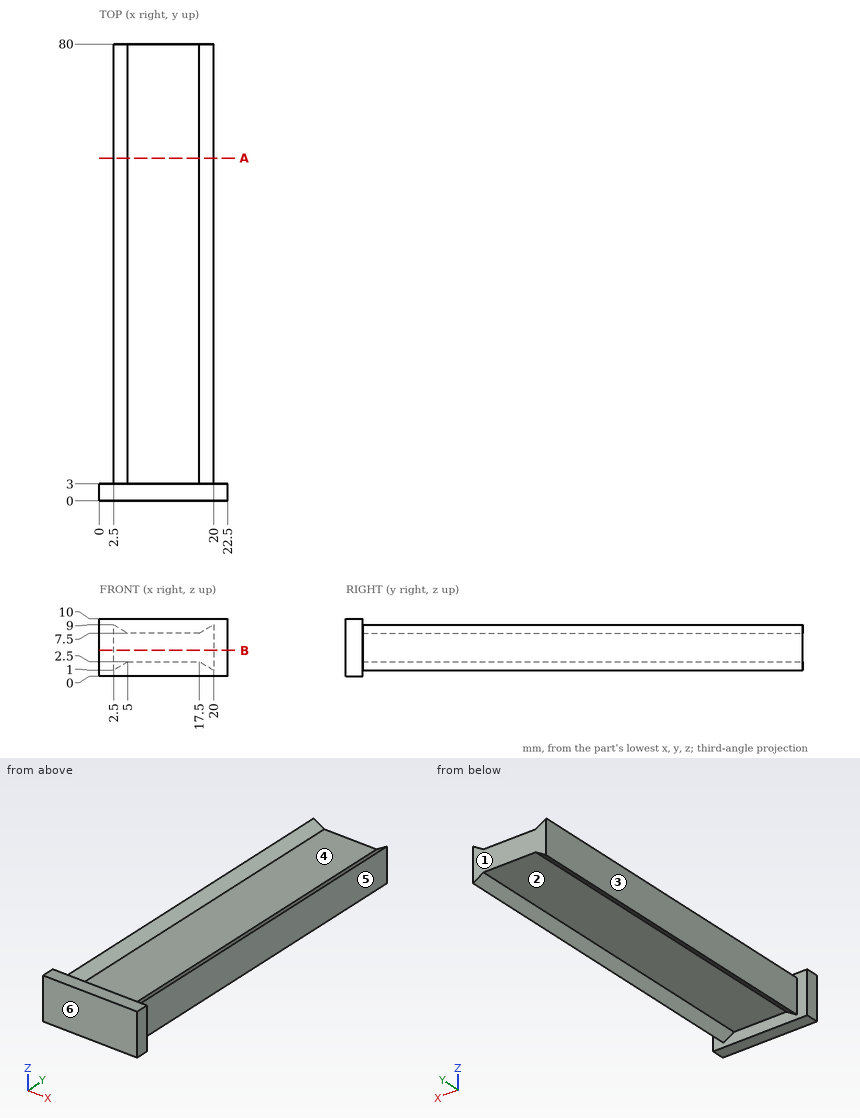
Geometry check sheet. Reference: drawing and pictorial views, mm from the part's lowest x, y, z. A direction names the side the tool comes from. Give positions to 0.01 mm unless a question says otherwise; leave off trailing zeros. Order: outer loops, then holes, each group sorted by start corner. A loop starts at its lowest first (then second) coordinate and runs counter-clockwise, first axis right, second up. Notation, with made-up numbers: M -33.75,-18.75 L 3.25,-18.75 A8 cw 3.25,-8.75 Z; hole C 52.5,3 d6. An arc over 180 degrees is marked long. Answer in a Markdown table with one row per item. Add a question column.
Q1. Release check for a two-part mould opening along X. For the marked faces 1, 2, 3 and 4 record: released by +X, released by -X, zero draft, split by the parting line, or undercut.
Q2. Sectioned sample at A-A, the plane y = 60. Record the boundary of the cut face in (x, z), and give its area (3 significant figures).
Q3. Gauge pin test, flat ends, axial feed: pin 1 Ø6 at (y, z) = (65, 8) entering from -X; pin 2 Ø12 at (x, y) = (9, 50.5) entering from +Z; pin 3 Ø6 at (x, y) = (9, 31) entering from -Z. Record the tip position at first contact, or that the pin passes through.
Q4. Sectioned sample at B-B, the plane z = 4.5. Record the boundary of the cut face in (x, y), and give its area (4 significant figures).
Q5. Thickness scan on L1, parallel to X at y = 6.5, z = 6.5; L2, parallel to Z at x = 7.75, y = 42; L3, parallel to Y at x = 12.5, z = 8.5. Record the ranges inside material, lowest first.
Q6. Access from +Z, -Z, +X, -X, +Y, -Y to the whole of each face (thin tool, end or side, straight path). Record for the marked faces 5 and 6.
Verdict:
| question | item | result |
|---|---|---|
| 1 | face 1 | zero draft |
| 1 | face 2 | undercut |
| 1 | face 3 | released by -X |
| 1 | face 4 | undercut |
| 2 | outline | M 2.5,1 L 5,2.5 L 17.5,2.5 L 20,1 L 20,9 L 17.5,7.5 L 5,7.5 L 2.5,9 Z |
| 2 | area | 95.0 mm² |
| 3 | pin 1 | x = 2.5 |
| 3 | pin 2 | z = 8.7 |
| 3 | pin 3 | z = 2.5 |
| 4 | outline | M 0,0 L 22.5,0 L 22.5,3 L 20,3 L 20,80 L 2.5,80 L 2.5,3 L 0,3 Z |
| 4 | area | 1,415 mm² |
| 5 | L1 | 2.5 to 20 |
| 5 | L2 | 2.5 to 7.5 |
| 5 | L3 | 0 to 3 |
| 6 | face 5 | +Z, -Z, +X, +Y |
| 6 | face 6 | +Z, -Z, +X, -X, -Y |
